from build123d import *

# Parameters (mm, degrees)
BOX003_W               = 2
BOX003_H               = 19
BOX003_DEPTH           = 25
BOX003_PLACEMENT_ANGLE = -90
BOX002_W               = 2
BOX002_H               = 8
BOX002_DEPTH           = 25
BOX001_W               = 2
BOX001_H               = 13
BOX001_DEPTH           = 25
BOX001_PLACEMENT_ANGLE = -90
BOX_W                  = 2
BOX_H                  = 45
BOX_DEPTH              = 25
FILLET006_R            = 1.5
FILLET007_R            = 1


with BuildPart() as box003:
    # Box003 → Box003 (new body)
    with BuildSketch(Plane.XY):
        with Locations((1, 9.5)):
            Rectangle(BOX003_W, BOX003_H)
    extrude(amount=BOX003_DEPTH)


with BuildPart() as box003_1:
    # Box003 placement: moved
    add(box003.part.moved(Location((10, 55, 0))).rotate(Axis((10, 55, 0), (0, 0, 1)), BOX003_PLACEMENT_ANGLE))


with BuildPart() as box002:
    # Box002 → Box002 (new body)
    with BuildSketch(Plane(origin=(10, 45, 0), x_dir=(1, 0, 0), z_dir=(0, 0, 1))):
        with Locations((1, 4)):
            Rectangle(BOX002_W, BOX002_H)
    extrude(amount=BOX002_DEPTH)


with BuildPart() as box001:
    # Box001 → Box001 (new body)
    with BuildSketch(Plane.XY):
        with Locations((1, 6.5)):
            Rectangle(BOX001_W, BOX001_H)
    extrude(amount=BOX001_DEPTH)


with BuildPart() as box001_1:
    # Box001 placement: moved
    add(box001.part.moved(Location((-1, 45, 0))).rotate(Axis((-1, 45, 0), (0, 0, 1)), BOX001_PLACEMENT_ANGLE))


with BuildPart() as obj1:
    # Box → Box (new body)
    with BuildSketch(Plane(origin=(-2, 0, 0), x_dir=(1, 0, 0), z_dir=(0, 0, 1))):
        with Locations((1, 22.5)):
            Rectangle(BOX_W, BOX_H)
    extrude(amount=BOX_DEPTH)

    # Fusion: union Box001
    add(box001_1.part)

    # Fusion001: union Box003, Box002
    add(box003_1.part)
    add(box002.part)

    # Fillet006
    fillet006_edges = [obj1.edges().sort_by_distance(p)[0] for p in [
        (-2, 45, 12.5),
        (10, 45, 12.5),
        (0, 43, 12.5),
        (12, 43, 12.5),
        (10, 55, 12.5),
        (12, 53, 12.5),
    ]]
    fillet(fillet006_edges, radius=FILLET006_R)

    # Fillet007
    fillet007_edges = [obj1.edges().sort_by_distance(p)[0] for p in [
        (-1, 0, 25),
        (-1, 0, 0),
    ]]
    fillet(fillet007_edges, radius=FILLET007_R)


solid = obj1.part
Verification items for the finished model (mm, model axes). A direction names the side the tool comes from. Give positions to 0.01 mm unless a question says otherwise; leave off trailing zeros. Loops run counter-clockwise (first coordinate to the right, second up) from the corner with the lowest first, then second, coordinate; pieces in that order, holes last.
1) Sectioned sample at A-A, the plane z = 8.5. Enter the section's corners in (x, y).
2) Depth check by flat-ended pin: pin 1 Ø6 at (y, z) = (27.5, 11) entering from +X; pin 2 Ø5.5 at (y, z) = (51, 12) entering from -X; pin 3 Ø2.5 at (x, z) = (5, 14) entering from -Y. Enter the tip coordinate at first touch or a pass-through.
3) Sectioned sample at B-B, the plane x = 6. Enter the section's corners in (y, z), then the cut area to 3 significant figures.
4) Thickness scan on line 1 along Y through (x, z) = (3, 20.25); line 2 along X through (y, z) = (14, 15.5); line 3 along Y through (x, z) = (19, 1.25). Record the ranges inside material, lowest first.
5) Sectioned sample at C-C, the plane y = 20.5. Enter the section's corners in (x, z).
6) Set-up check for faces 1 (the flat face through (-0.4, 34.1, 0)), 2 (the flat face through (10, 50, 12)), 3 (the flat face through (21, 53, 12)): record each of +Z, -Z, +X, -X, +Y, -Y from which the full face is reachable in a straight line by a thin tool's end or side.
Answers:
1. outline: (-2, 0) - (0, 0) - (0, 41.5) arc R1.5 cw to (1.5, 43) - (10.5, 43) arc R1.5 ccw to (12, 44.5) - (12, 51.5) arc R1.5 cw to (13.5, 53) - (29, 53) - (29, 55) - (11.5, 55) arc R1.5 ccw to (10, 53.5) - (10, 46.5) arc R1.5 cw to (8.5, 45) - (-0.5, 45) arc R1.5 ccw to (-2, 43.5) - close
2. pin 1: stops at x = 0
2. pin 2: stops at x = 10
2. pin 3: stops at y = 43
3. outline: (43, 0) - (45, 0) - (45, 25) - (43, 25) - close
3. area: 50.0 mm2
4. line 1: y = 43 to 45
4. line 2: x = -2 to 0
4. line 3: y = 53 to 55
5. outline: (-2, 0) - (0, 0) - (0, 25) - (-2, 25) - close
6. face 1: -Z, +X, -X, +Y, -Y
6. face 2: +Z, -Z, -X, +Y
6. face 3: +Z, -Z, +X, -Y
